```python
from build123d import *


with BuildPart() as f1:
    # F0 (on Right) → F1 (revolve)
    with BuildSketch(Plane.YZ):
        with BuildLine():
            Line((-2, 1.504770412), (-2, 0))
            Line((-2, 0), (9.5, 0))
            add(Edge.make_bspline(
                [(8, 2.45), (8.6955977604, 2.2305608727), (9.2895837523, 1.318056569), (9.4629809577, 0.4408934937), (9.5, 0)],
                knots=[0, 0, 0, 0, 0.532645082, 1, 1, 1, 1], degree=3))
            Line((8, 2.45), (1, 2.45))
            Line((1, 2.45), (1, 4.004770412))
            Line((1, 4.004770412), (0, 4.004770412))
            Line((0, 4.004770412), (0, 1.504770412))
            Line((0, 1.504770412), (-2, 1.504770412))
        make_face()
    revolve(axis=Axis((0, 3.75, 0), (0, -1, 0)))


solid = f1.part
```
Geometry: final body of the model. Coordinates: model frame, mm. A direction names the side the tool comes from. Round coordinates to 2 decimals unless told otherwise and drop trailing zeros. Loops run counter-clockwise (first coordinate to the right, second up) from the corner with the lowest first, then second, coordinate; pieces in that order, holes last. Notation, with made-up numbers: (88, 89.5) -> (123, 89.5) arc R8 ccw to (123, 98.5) -> close; hole circle Ø5 at (82, 58.5). An arc over 180 degrees is marked (long way). Write each question's results on one line, items separated by ' | '.
Item 1: Cut plane A-A on y = 2.5. Return the cut outline in (x, z).
Answers below:
outline: circle Ø4.9 at (0, 0)
Item 2: Set-up query: faces 1 (the face through (-2, 1, -2)), 2 (the face through (0, -2, 0)), 3 (the face through (0.92, -1.01, -1.19)). Return all of +Z, -Z, +X, -X, +Y, -Y with unobstructed straight access to the full face (end or side cutting, diameter ignored); none if empty.
Answers below:
face 1: +Y | face 2: +Z, -Z, +X, -X, -Y | face 3: -Y
Item 3: Pin query (flat end, axial travel): pin 1 Ø2 at (x, z) = (-2, -3) entering from -Y; pin 2 Ø2 at (x, y) = (-3, 5.5) entering from +Z; pin 3 Ø3 at (x, y) = (0.5, 5.5) entering from -Z. Return the tip coordinate at first contact, or that it passes through.
Answers below:
pin 1: stops at y = 0 | pin 2: stops at z = 1.42 | pin 3: stops at z = -2.45
Item 4: Line query: probe 1 along Y at (x, z) = (-3.5, -1); probe 2 along X at (y, z) = (6, 0); probe 3 along X at (y, z) = (7.75, -2.25). Output: solid intervals per line, ascending. Write a range as [from, to].
Answers below:
probe 1: y = [0, 1] | probe 2: x = [-2.45, 2.45] | probe 3: x = [-0.97, 0.97]
Item 5: Cut plane C-C on x = -3.5. Return the cut outline in (y, z), and give its area (3 significant figures).
Answers below:
outline: (0, -1.95) -> (1, -1.95) -> (1, 1.95) -> (0, 1.95) -> close | area: 3.89 mm²
Item 6: Cut plane B-B on z = 3. Return the cut outline in (x, y), and give its area (3 significant figures).
Answers below:
outline: (-2.65, 0) -> (2.65, 0) -> (2.65, 1) -> (-2.65, 1) -> close | area: 5.31 mm²
